Autodesk Inventor part; units mm, degrees
ref_plane "YZ Plane" through (0, 0, 0) normal (1, 0, 0) x (0, 1, 0)
ref_plane "XZ Plane" through (0, 0, 0) normal (0, 1, 0) x (-1, 0, 0)
ref_plane "XY Plane" through (0, 0, 0) normal (0, 0, 1) x (1, 0, 0)
sketch "Esquisse1" plane through (0, 0, 0) normal (0, 0, 1) x (1, 0, 0)
  line L0 (7.5, 0) -> (-7.5, 0)
  line L1 (-7.5, 0) -> (-7.5, 11.5)
  line L2 (-7.5, 11.5) -> (7.5, 11.5)
  line L3 (7.5, 11.5) -> (7.5, 0)
  point P0 (0, 0)
  dimension "d0" = 15
  dimension "d1" = 11.5
  dimension "d2" = 0
  dimension "d3" = 7.5
extrude "Extrusion1" add sketch "Esquisse1" along normal blind 17.5
sketch "Esquisse2" plane through (0, 0, 17.5) normal (0, 0, 1) x (1, 0, 0)
  line L0 (-7.5, 0) -> (7.5, 0)
  line L1 (7.5, 0) -> (7.5, 11.5)
  line L2 (7.5, 11.5) -> (-7.5, 11.5)
  line L3 (-7.5, 11.5) -> (-7.5, 0)
  line L4 (-6, 0) -> (6, 0)
  line L5 (6, 0) -> (6, 10)
  line L6 (6, 10) -> (-6, 10)
  line L7 (-6, 10) -> (-6, 0)
  point P0 (0, 0)
  dimension "d6" = 1.5
  dimension "d7" = 1.5
  dimension "d8" = 1.5
extrude "Extrusion2" cut sketch "Esquisse2" against normal through all contours L7 L6 L5 L0
fillet "Congé1" radius 1 2 edges at (7.5, 11.5, 8.75) (-7.5, 11.5, 8.75)
sketch "Esquisse4" plane through (7.5, 0, 0) normal (0, -1, 0) x (1, 0, 0)
  line L0 (0, 0) -> (0, 17.5)
  circle A0 centre (-16.25, 13.5) radius 1.25
  circle A1 centre (1.25, 13.5) radius 1.25
  line L1 (1.25, 9) -> (0, 9)
  line L2 (-16.25, 9) -> (-15, 9)
  line L3 (-16.25, 14.75) -> (-15, 14.75)
  line L4 (-16.25, 12.25) -> (-15, 12.25)
  line L5 (1.25, 14.75) -> (0, 14.75)
  line L6 (1.25, 12.25) -> (0, 12.25)
  line L7 (0, 12.25) -> (0, 9)
  line L8 (0, 17.5) -> (0, 14.75)
  line L9 (-15, 17.5) -> (-15, 14.75)
  line L10 (-15, 12.25) -> (-15, 9)
  arc A2 (-18.3116, 17.5) -> (-16.25, 9) centre (-16.25, 13.5) ccw
  line L11 (-13.5, 17.5) -> (-1.5, 17.5)
  arc A3 (1.25, 9) -> (3.3116, 17.5) centre (1.25, 13.5) ccw
  line L12 (-18.3116, 17.5) -> (-15, 17.5)
  line L13 (0, 17.5) -> (3.3116, 17.5)
  point P0 (-7.5, 0)
  dimension "d12" = 2.5
  dimension "d13" = 2.5
  dimension "d14" = 17.5
  dimension "d15" = 8.75
  dimension "d18" = 4
  dimension "d22" = 4.5
  dimension "d23" = 3.25
  dimension "d24" = 5.25
  dimension "d25" = 4.5
  dimension "d26" = 3.25
  dimension "d27" = 152.734
  dimension "d28" = 152.734
extrude "Extrusion5" add sketch "Esquisse4" against normal blind 3 contours L0 L6 A1 L5 L13 A3 L1 | A0 L4 L10 L2 A2 L12 L9 L3
fillet "Congé2" radius 1 4 edges at (-7.5, 3, 10.625) (-7.5, 3, 16.125) (7.5, 3, 16.125) (7.5, 3, 10.625)
properties part number "fixation moteur" material "Plastique ABS"
The model under review builds one solid part; all positions refer to its coordinate system, in mm. A direction names the side the tool comes from. Coordinates: 2 decimals unless noted, no trailing zeros. Order: outer loops, then holes, each group sorted by start corner. A loop starts at its lowest first (then second) coordinate and runs counter-clockwise, first axis right, second up. Notation, with made-up numbers: (74.25, -34) -> (125.25, -34) arc R25 cw to (125.25, 2) -> close; hole circle Ø5 at (42.5, 80.5). An arc over 180 degrees is marked (long way). Answer in a Markdown table with one row per item.
(1) Consider section D-D (x = -1.75). Write out the cut boundary in (y, z), plus the area to 4 significant figures.
Answers:
| item | result |
|---|---|
| outline | (10, 0) -> (11.5, 0) -> (11.5, 17.5) -> (10, 17.5) -> close |
| area | 26.25 mm² |
(2) Insertion check: pin 1 (1 mm diameter, centred on y = 9, z = 10.5, fed in from +X); pin 2 (1.4 mm diameter, centred on x = 11, z = 13.5, fed in from +Y); pin 3 (5 mm diameter, centred on y = 6.5, z = 11, fed in from -X). Each pin has a flat end and moves straight along its axis. Give the tip position at first contact, or say it passes through.
Answers:
| item | result |
|---|---|
| pin 1 | x = 7.5 |
| pin 2 | y = 3 |
| pin 3 | x = -7.5 |
(3) Consider section B-B (z = 13.5). Write out the cut boundary in (x, y).
Answers:
| item | result |
|---|---|
| outline | (-13.25, 0) -> (-10, 0) -> (-10, 3) -> (-13.25, 3) -> close; (-7.5, 0) -> (-6, 0) -> (-6, 10) -> (6, 10) -> (6, 0) -> (7.5, 0) -> (7.5, 10.5) arc R1 ccw to (6.5, 11.5) -> (-6.5, 11.5) arc R1 ccw to (-7.5, 10.5) -> close; (10, 0) -> (13.25, 0) -> (13.25, 3) -> (10, 3) -> close |
(4) The part is to be moulded in two halves that separate along Z. For faces 1 (the flat face through (-0.6, 10.5, 0)), 2 (the cylindrical face through (13.103, 1.479, 12.358)), 3 (the flat face through (8, 2, 14.75)), 4 (the cylindrical face through (-10, 1.5, 13.5)), say which applies: +Z half, -Z half, draft (parallel to the pull), parting line (faces both ways), or undercut.
Answers:
| item | result |
|---|---|
| face 1 | -Z half |
| face 2 | parting line |
| face 3 | undercut |
| face 4 | undercut |
(5) Consider section A-A (y = 7.75). Write out the cut boundary in (x, z).
Answers:
| item | result |
|---|---|
| outline | (-7.5, 0) -> (-6, 0) -> (-6, 17.5) -> (-7.5, 17.5) -> close; (6, 0) -> (7.5, 0) -> (7.5, 17.5) -> (6, 17.5) -> close |
(6) Wall thickness on line 1 along X through (y, z) = (1.5, 8.5); line 2 along X through (y, z) = (10.5, 9.5); line 3 along Y through (x, z) = (0.25, 4): over which ranges is each line inside the solid? List them lowest first.
Answers:
| item | result |
|---|---|
| line 1 | -7.5 to -6, 6 to 7.5 |
| line 2 | -7.5 to 7.5 |
| line 3 | 10 to 11.5 |
(7) Machinability: for faces 5 (the flat face through (8, 2, 9)), 6 (the flat face through (-8, 2, 9)), 7 (the flat face through (6, 5, 9)), which of the approach directions +Z, -Z, +X, -X, +Y, -Y give a long, thin tool a straight path to every point of the face, cutting with its end or side? Answer none if there is none.
Answers:
| item | result |
|---|---|
| face 5 | -Z, +X, +Y, -Y |
| face 6 | -Z, -X, +Y, -Y |
| face 7 | +Z, -Z, -Y |
(8) Consider section C-C (z = 1.5). Write out the cut boundary in (x, y), plus the area to 3 significant figures.
Answers:
| item | result |
|---|---|
| outline | (-7.5, 0) -> (-6, 0) -> (-6, 10) -> (6, 10) -> (6, 0) -> (7.5, 0) -> (7.5, 10.5) arc R1 ccw to (6.5, 11.5) -> (-6.5, 11.5) arc R1 ccw to (-7.5, 10.5) -> close |
| area | 52.1 mm² |
